The listing builds one solid part. Answer for the finished solid, in the listing's coordinates (mm). A direction names the side the tool comes from. Coordinates: 2 decimals unless noted, no trailing zeros. Loops run counter-clockwise (first coordinate to the right, second up) from the corner with the lowest first, then second, coordinate; pieces in that order, holes last. Notation, with made-up numbers: (59.25, 61.5) -> (100.25, 61.5) arc R21 ccw to (100.25, 83.5) -> close; hole circle Ø4 at (32.5, 31.25). An arc over 180 degrees is marked (long way). Answer in a Markdown table with one row per item.
```python
from build123d import *

# Parameters (mm, degrees)
F1_DEPTH  = 18.5
F3_DEPTH  = 54
F5_DEPTH  = 48.5
F6_R      = 5
F7_DEPTH  = 65.001
F8_W      = 12
F8_H      = 12
F9_DEPTH  = 8
F10_W     = 71
F10_H     = 2
F11_DEPTH = 11
F13_DEPTH = 11.001
F17_R     = 6


# Not quite as in the source:
# - a pattern or mirror of a feature is missing from the dataset's text; its kind, count and spacing are read off the source's solid


with BuildPart() as f1:
    # F0 (on Front) → F1 (new body, symmetric)
    with BuildSketch(Plane.XZ):
        Polygon((-82, 11), (-85, 0), (85, 0), (82, 11), align=None)
    extrude(amount=F1_DEPTH, both=True)

    # F2 (on face) → F3 (join)
    with BuildSketch(Plane.XY.offset(11)):
        with BuildLine():
            Line((38.8168777724, 18.5), (-38.8168777724, 18.5))
            ThreePointArc((-38.8168777724, 18.5), (-43, 0), (-38.8168777724, -18.5))
            Line((-38.8168777724, -18.5), (38.8168777724, -18.5))
            ThreePointArc((38.8168777724, -18.5), (43, 0), (38.8168777724, 18.5))
        make_face()
    extrude(amount=F3_DEPTH)

    # F4 (on Front) → F5 (cut, symmetric)
    with BuildSketch(Plane.XZ):
        with BuildLine():
            Line((22, 65), (-22, 65))
            Line((-22, 65), (-22, 52))
            Line((-22, 52), (-19, 52))
            Line((-19, 52), (-19, 49))
            ThreePointArc((-19, 49), (0, 30), (19, 49))
            Line((19, 49), (19, 52))
            Line((19, 52), (22, 52))
            Line((22, 52), (22, 65))
        make_face()
    extrude(amount=F5_DEPTH, both=True, mode=Mode.SUBTRACT)

    # F6 (on face) → F7 (cut, through all)
    with BuildSketch(Plane.XY.offset(65)):
        with Locations((-31, 0)):
            Circle(F6_R)
        with Locations((31, 0)):
            Circle(F6_R)
    extrude(amount=-F7_DEPTH, mode=Mode.SUBTRACT)

    # F8 (on face) → F9 (cut)
    with BuildSketch(Plane(origin=(0, 0, 0), x_dir=(1, 0, 0), z_dir=(0, 0, -1))):
        with Locations((-31, 0)):
            Rectangle(F8_W, F8_H)
        with Locations((31, 0)):
            Rectangle(F8_W, F8_H)
    extrude(amount=-F9_DEPTH, mode=Mode.SUBTRACT)

    # F10 (on Front) → F11 (cut, symmetric)
    with BuildSketch(Plane.XZ):
        with Locations((-39.5, 1)):
            Rectangle(F10_W, F10_H)
    f11 = extrude(amount=F11_DEPTH, both=True, mode=Mode.SUBTRACT)

    # F11_copies: F11 across plane
    add(f11.mirror(Plane(origin=(0, 0, 0), x_dir=(0, 0, 1), z_dir=(1, 0, 0))), mode=Mode.SUBTRACT)

    # F12 (on face) → F13 (cut, through all)
    with BuildSketch(Plane.XY.offset(11)):
        with BuildLine():
            ThreePointArc((-70, 5), (-75, 0), (-70, -5))
            Line((-70, -5), (-64, -5))
            ThreePointArc((-64, -5), (-59, 0), (-64, 5))
            Line((-64, 5), (-70, 5))
        make_face()
        with BuildLine():
            ThreePointArc((70, -5), (75, 0), (70, 5))
            Line((70, 5), (64, 5))
            ThreePointArc((64, 5), (59, 0), (64, -5))
            Line((64, -5), (70, -5))
        make_face()
    extrude(amount=-F13_DEPTH, mode=Mode.SUBTRACT)

    # F14 (on Front) → F15 (revolve, cut)
    with BuildSketch(Plane.XZ):
        Polygon((3, 31.8085759505), (0, 31.8085759505), (0, 22.1974181429), (3, 24), align=None)
    revolve(axis=Axis((0, 0, 27.0029970467), (0, 0, -1)), mode=Mode.SUBTRACT)

    # F14 (on Front) → F16 (revolve, cut)
    with BuildSketch(Plane.XZ):
        Polygon((3, 31.8085759505), (0, 31.8085759505), (0, 22.1974181429), (3, 24), align=None)
    revolve(axis=Axis((0, 0, 27.0029970467), (0, 0, -1)), mode=Mode.SUBTRACT)

    # F17
    f17_edges = [f1.edges().sort_by_distance(p)[0] for p in [
        (43, 0, 11),
        (-43, 0, 11),
    ]]
    fillet(f17_edges, radius=F17_R)


solid = f1.part
```
Item 1: A cutting plane is placed at C-C, the plane x = 9.5. Determine the outline of the cut face in (y, z).
Findings below:
| item | result |
|---|---|
| outline | (-18.5, 0) -> (-11, 0) -> (-11, 2) -> (11, 2) -> (11, 0) -> (18.5, 0) -> (18.5, 32.55) -> (-18.5, 32.55) -> close |
Item 2: A tool of negligible diameter and unlimited length cuts with its end or side. For faces 4 (the face through (-67, -5, 7)), 5 (the face through (-25.8, -0.1, 8)), 6 (the face through (-19, 0, 51)), from which of +Z, -Z, +X, -X, +Y, -Y can it reach the whole face along a straight path? Write none if from no direction.
Findings below:
| item | result |
|---|---|
| face 4 | +Z, -Z |
| face 5 | -Z |
| face 6 | +Z, +Y, -Y |
Item 3: A cutting plane is placed at B-B, the plane x = -31. Determine the outline of the cut face in (y, z), plus the area to 3 significant figures.
Findings below:
| item | result |
|---|---|
| outline | (-18.5, 0) -> (-11, 0) -> (-11, 2) -> (-6, 2) -> (-6, 8) -> (-5, 8) -> (-5, 65) -> (-18.5, 65) -> close; (5, 8) -> (6, 8) -> (6, 2) -> (11, 2) -> (11, 0) -> (18.5, 0) -> (18.5, 65) -> (5, 65) -> close |
| area | 1,720 mm2 |
Item 4: Flat-ended cylindrical pins translate along their axes: pin 1 Ø1.8 at (y, z) = (-2.5, 3.5) entering from -X; pin 2 Ø8 at (y, z) = (1.5, 42) entering from -X; pin 3 Ø3 at (y, z) = (-0.5, 6) entering from +X. Find the tip coordinate at first contact, or state that the pin passes through.
Findings below:
| item | result |
|---|---|
| pin 1 | stops at x = -84.29 |
| pin 2 | stops at x = -43 |
| pin 3 | stops at x = 83.77 |
Item 5: Find the intervals of material crossed by probe 1 along Y at (x, z) = (0, 26.5); probe 2 along Y at (x, z) = (31, 51); probe 3 along Z at (x, y) = (51, 14.5), in increasing order.
Findings below:
| item | result |
|---|---|
| probe 1 | y = -18.5 to -3, 3 to 18.5 |
| probe 2 | y = -18.5 to -5, 5 to 18.5 |
| probe 3 | z = 0 to 11 |
Item 6: A cutting plane is placed at D-D, the plane x = 30.5. Determine the outline of the cut face in (y, z), plus the area to 3 significant figures.
Findings below:
| item | result |
|---|---|
| outline | (-18.5, 0) -> (-11, 0) -> (-11, 2) -> (-6, 2) -> (-6, 8) -> (-4.97, 8) -> (-4.97, 65) -> (-18.5, 65) -> close; (4.97, 8) -> (6, 8) -> (6, 2) -> (11, 2) -> (11, 0) -> (18.5, 0) -> (18.5, 65) -> (4.97, 65) -> close |
| area | 1,720 mm2 |
Item 7: A cutting plane is placed at A-A, the plane z = 41. Determine the outline of the cut face in (x, y).
Findings below:
| item | result |
|---|---|
| outline | (-38.82, -18.5) -> (-17.23, -18.5) -> (-17.23, 18.5) -> (-38.82, 18.5) arc R43 ccw to start; (17.23, -18.5) -> (38.82, -18.5) arc R43 ccw to (38.82, 18.5) -> (17.23, 18.5) -> close; hole circle Ø10 at (-31, 0); hole circle Ø10 at (31, 0) |
Item 8: Determine the mould class of faces 1 (the face through (-25, 0, 5)), 2 (the face through (43, 0, 41)), 3 (the face through (-1, 18.5, 19)) for opening direction X: +X half, -X half, draft (parallel to the pull), parting line (faces both ways), or undercut.
Findings below:
| item | result |
|---|---|
| face 1 | undercut |
| face 2 | +X half |
| face 3 | draft |
